Geometry: final body of the model. Coordinates: model frame, mm. A direction names the side the tool comes from. Give positions to 0.01 mm unless a question says otherwise; leave off trailing zeros. Write each loop counter-clockwise with the first axis right and the second up, starting at its lowest first coordinate (ties: lowest second). Pieces come first, ordered by that corner, then holes.
from build123d import *
from build123d.topology import SkipClean

# Parameters (mm, degrees)
SKETCH_1_R              = 5.5
EXTRUDE_1_DEPTH         = 18
SKETCH_2_R              = 4
CUT_EXTRUDE_1_DEPTH     = 18
EXTRUDE_2_DEPTH         = 18
CUT_EXTRUDE_3_DEPTH     = 6
EXTRUDE_START           = 6
EXTRUDE_3_DEPTH         = 6
SKETCH_11_R             = 5.5
EXTRUDE_4_DEPTH         = 7
EXTRUDE_START_2         = 2
SKETCH_15_R             = 5.5
EXTRUDE_5_DEPTH         = 2
HOLE_WIZARD_M4_4_D      = 3.3
CUT_EXTRUDE_8_DEPTH     = 8
SKETCH_20_W             = 0.38
SKETCH_20_H             = 4
CUT_EXTRUDE_9_DEPTH     = 8
HOLE_WIZARD_M4_9_D      = 3.3
HOLE_WIZARD_M4_9_DEPTH  = 2
HOLE_WIZARD_M4_10_D     = 3.3
HOLE_WIZARD_M4_10_DEPTH = 1.5
CHAMFER_2_SIZE          = 0.2
CHAMFER_3_SIZE          = 0.2


with BuildPart() as part:
    # 草图1 → 凸台-拉伸1 (new body)
    with BuildSketch(Plane.XY):
        Circle(SKETCH_1_R)
    extrude(amount=EXTRUDE_1_DEPTH)

    # 草图2 → 切除-拉伸1 (cut)
    with BuildSketch(Plane(origin=(0, 0, 0), x_dir=(-1, 0, 0), z_dir=(0, 0, -1))):
        Circle(SKETCH_2_R)
    extrude(amount=-CUT_EXTRUDE_1_DEPTH, mode=Mode.SUBTRACT)

    # 草图3 → 凸台-拉伸2 (add)
    with BuildSketch(Plane(origin=(0, 0, 0), x_dir=(-1, 0, 0), z_dir=(0, 0, -1))):
        Polygon((-3.5, 0), (-3.5, 2.515567), (-4.944421, -0.303566), (-4.222211, -2.180275), (-3.5, -2.180275), align=None)
    extrude(amount=-EXTRUDE_2_DEPTH)

    # 草图5 → 切除-拉伸3 (cut)
    with BuildSketch(Plane(origin=(0, 0, 0), x_dir=(-1, 0, 0), z_dir=(0, 0, -1))):
        Polygon((-4.5, 0), (-4.5, -1.5), (-5.291503, -1.5), (-6.679987, 0.400671), (-5.291503, 1.5), (-4.5, 1.5), align=None)
    extrude(amount=-CUT_EXTRUDE_3_DEPTH, mode=Mode.SUBTRACT)

    # 草图6 → 凸台-拉伸3 (add)
    with SkipClean():  # the faces are left unmerged after this step: merging them gives an invalid solid
        with BuildSketch(Plane(origin=(0, 0, 6), x_dir=(-1, 0, 0), z_dir=(0, 0, -1)).offset(EXTRUDE_START)):
            with BuildLine():
                Line((-5.291503, -1.5), (-4.238481, -1.644386))
                Line((-4.238481, -1.644386), (-3.814049, 1.930313))
                Line((-3.814049, 1.930313), (-5.291503, 1.5))
                ThreePointArc((-5.291503, 1.5), (-5.5, 0), (-5.291503, -1.5))
            make_face()
        extrude(amount=-EXTRUDE_3_DEPTH)

    # 草图11 → 凸台-拉伸4 (add)
    with SkipClean():  # the faces are left unmerged after this step: merging them gives an invalid solid
        with BuildSketch(Plane.XY.offset(18)):
            Circle(SKETCH_11_R)
        extrude(amount=EXTRUDE_4_DEPTH)

    # 草图15 → 凸台-拉伸5 (add)
    with SkipClean():  # the faces are left unmerged after this step: merging them gives an invalid solid
        with BuildSketch(Plane(origin=(0, 0, 18), x_dir=(-1, 0, 0), z_dir=(0, 0, -1)).offset(EXTRUDE_START_2)):
            with Locations(Location((0, 0, 0), (0, 0, 180))):
                Circle(SKETCH_15_R)
        extrude(amount=-EXTRUDE_5_DEPTH)

    # M4 螺纹孔4 (through all)
    with Locations(Plane.XY.offset(25)):
        with Locations((0, 0)):
            Hole(HOLE_WIZARD_M4_4_D / 2)

    # 草图19 → 切除-拉伸8 (cut)
    with SkipClean():  # the faces are left unmerged after this step: merging them gives an invalid solid
        with BuildSketch(Plane.XY.offset(25)):
            Polygon((-5.5, 0), (-5.5, -2), (-3.5, -2), (-3.5, 2), (-5.5, 2), align=None)
        extrude(amount=-CUT_EXTRUDE_8_DEPTH, mode=Mode.SUBTRACT)

    # 草图20 → 切除-拉伸9 (cut)
    with SkipClean():  # the faces are left unmerged after this step: merging them gives an invalid solid
        with BuildSketch(Plane.XY.offset(25)):
            with Locations((-3.31, 0)):
                Rectangle(SKETCH_20_W, SKETCH_20_H)
        extrude(amount=-CUT_EXTRUDE_9_DEPTH, mode=Mode.SUBTRACT)

    # M4 螺纹孔9
    with Locations(Plane(origin=(3.5, 0, 6), x_dir=(0, 0, -1), z_dir=(-1, 0, 0))):
        with Locations((0, 0)):
            Hole(HOLE_WIZARD_M4_9_D / 2, depth=HOLE_WIZARD_M4_9_DEPTH)

    # M4 螺纹孔10
    with Locations(Plane(origin=(-0.112691, 3.998412, 5.952809), x_dir=(-0.999603066556, -0.028172847433, 0), z_dir=(0.028172847433, -0.999603066556, 0))):
        with Locations((0, 0)):
            Hole(HOLE_WIZARD_M4_10_D / 2, depth=HOLE_WIZARD_M4_10_DEPTH)

    # 倒角2
    chamfer_2_edges = [part.edges().sort_by_distance(p)[0] for p in [
        (1.017567, 5.405049, 25),
    ]]
    chamfer(chamfer_2_edges, length=CHAMFER_2_SIZE)

    # 倒角3
    chamfer_3_edges = [part.edges().sort_by_distance(p)[0] for p in [
        (-5.291503, -1.5, 0),
    ]]
    chamfer(chamfer_3_edges, length=CHAMFER_3_SIZE)


solid = part.part
Q1. Section A-A on y = 0. Output: boundary loops of the cut face in (x, z).
Filled sheet:
outline: (-5.5, 0.2) - (-5.3, 0) - (-4, 0) - (-4, 16) - (-1.65, 16) - (-1.65, 25) - (-3.12, 25) - (-3.12, 17) - (-5.5, 17) - close; (1.65, 16) - (3.5, 16) - (3.5, 7.65) - (5.5, 7.65) - (5.5, 24.8) - (5.3, 25) - (1.65, 25) - close; (3.5, 0) - (5.3, 0) - (5.5, 0.2) - (5.5, 4.35) - (3.5, 4.35) - close
Q2. Pin query (flat end, axial travel): P1, Ø1, axis at y = 2, z = 9, coming from the -X side; P2, Ø0.6, axis at x = -4, z = 19.5, coming from the +Y side; P3, Ø2.5, axis at x = -1, y = -1.5, coming from the -Z side; P4, Ø1.5, axis at x = 0.5, z = 22, coming from the -Y side. Return the tip coordinate at first contact, or that it passes through.
Filled sheet:
P1: stops at x = -5.29
P2: stops at y = 4.07
P3: stops at z = 16
P4: stops at y = -5.5
Q3. Section C-C on x = 0. Count the separate pieces of the cut face and the enclosed holes in it, plus the area to 3 significant figures.
Filled sheet:
separate pieces: 3
enclosed holes: 0
area: 112 mm2
Q4. Section B-B on z = 6.5. Output: boundary loops of the cut face in (x, y), plus the area to 3 significant figures.
Filled sheet:
outline: (-1.7, 5.23) arc R5.5 ccw (long way) to (5.27, -1.57) - (3.5, -1.57) - (3.5, -1.94) arc R4 cw (long way) to (-1.66, 3.64) - close; (1.41, 5.32) - (1.45, 3.73) arc R4 cw to (3.5, 1.94) - (3.5, 1.57) - (5.27, 1.57) arc R5.5 ccw to start
area: 35.3 mm2
Q5. Ray query, line 1 along Y through (x, z) = (0, 19); line 2 along X through (y, z) = (0, 9.5); line 3 along Z through (x, y) = (-2, 2). Return the intervals inside material, ascending.
Filled sheet:
line 1: y = -5.5 to -1.65, 1.65 to 5.5
line 2: x = -5.5 to -4, 3.5 to 5.5
line 3: z = 16 to 25
Q6. Pull-direction query (Y, two-part tool) for faces 4 (the flat face through (3.5, 0, 8)), 5 (the flat face through (1.3, 1.3, 25)); classes: released by +Y, released by -Y, zero draft, split by the parting line, or undercut.
Filled sheet:
face 4: undercut
face 5: zero draft
Q7. Access query for faces 1 (the cylindrical face through (1.394, 4.626, 6.585)), 2 (the flat face through (-3.12, 0, 21)), 3 (the cylindrical face through (-4, 0, 8)). Directions: +Z, -Z, +X, -X, +Y, -Y. A direction counts if a zero-diameter tool reaches every point of the face in a straight line with its end or side. Return the directions, or none.
Filled sheet:
face 1: none
face 2: +Z, -X
face 3: -Z
